from build123d import *

# Parameters (mm, degrees)
SKETCH_1_W          = 50
SKETCH_1_H          = 30
EXTRUDE_1_DEPTH     = 15
SKETCH_2_W          = 19
SKETCH_2_H          = 11.7
CUT_EXTRUDE_1_DEPTH = 28
SKETCH_4_W          = 7.5
SKETCH_4_H          = 13
CUT_EXTRUDE_3_DEPTH = 50
SKETCH_5_W          = 7.5
SKETCH_5_H          = 13
CUT_EXTRUDE_4_DEPTH = 50
CUT_EXTRUDE_5_DEPTH = 50


with BuildPart() as part:
    # Эскиз1 → Бобышка-Вытянуть1 (new body)
    with BuildSketch(Plane.XY):
        Rectangle(SKETCH_1_W, SKETCH_1_H)
    extrude(amount=EXTRUDE_1_DEPTH)

    # Эскиз2 → Вырез-Вытянуть1 (cut)
    with BuildSketch(Plane(origin=(0, 15, 0), x_dir=(1, 0, 0), z_dir=(0, 1, 0))):
        with Locations((0, -9.15)):
            Rectangle(SKETCH_2_W, SKETCH_2_H)
    extrude(amount=-CUT_EXTRUDE_1_DEPTH, mode=Mode.SUBTRACT)

    # Эскиз4 → Вырез-Вытянуть3 (cut)
    with BuildSketch(Plane(origin=(0, 15, 0), x_dir=(1, 0, 0), z_dir=(0, 1, 0))):
        with Locations((-21.25, -6.5)):
            Rectangle(SKETCH_4_W, SKETCH_4_H)
    extrude(amount=-CUT_EXTRUDE_3_DEPTH, mode=Mode.SUBTRACT)

    # Эскиз5 → Вырез-Вытянуть4 (cut)
    with BuildSketch(Plane(origin=(0, 15, 0), x_dir=(1, 0, 0), z_dir=(0, 1, 0))):
        with Locations((21.25, -6.5)):
            Rectangle(SKETCH_5_W, SKETCH_5_H)
    extrude(amount=-CUT_EXTRUDE_4_DEPTH, mode=Mode.SUBTRACT)

    # Эскиз6 → Вырез-Вытянуть5 (cut)
    with BuildSketch(Plane.XZ.offset(15)):
        with BuildLine():
            Line((-5, 15), (5, 15))
            ThreePointArc((5, 15), (0, 10), (-5, 15))
        make_face()
    extrude(amount=-CUT_EXTRUDE_5_DEPTH, mode=Mode.SUBTRACT)


solid = part.part
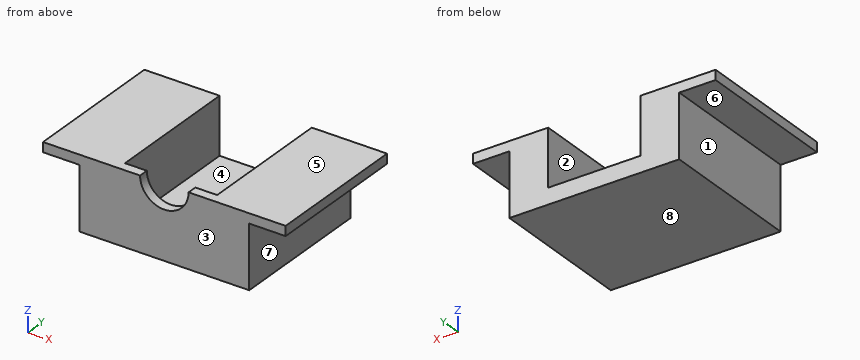
Here's how the part is built. I have some questions about the finished solid (model axes, mm). Face numbers are marked on the shaded views. A direction names the side the tool comes from. Coordinates: 2 decimals unless noted, no trailing zeros. Loops run counter-clockwise (first coordinate to the right, second up) from the corner with the lowest first, then second, coordinate; pieces in that order, holes last. Notation, with made-up numbers: (10.5, 36) -> (26.5, 36) arc R8 ccw to (26.5, 41) -> close; hole circle Ø4 at (-2.75, -4.5). An arc over 180 degrees is marked (long way). Use one line per item in the form item = value. Start each with the question number.
(1) If we section it at A-A (z = 9.25): Please give me the cut outline in (x, y).
(2) Please list where these lines run through material, in increasing order: line 1 along X through (y, z) = (4, 7); line 2 along Y through (x, z) = (6, 13.5); line 3 along Z through (x, y) = (2.5, -3.75).
(3) If we section it at B-B (x = 6): Please give me the cut outline in (y, z).
(4) We'd pull the mould along X, two halves only. Please class the marked faces 1, 2 and 3: pulls with the +X half, pulls with the -X half, needs draft (parallel to the pull), parting line crosses it, or undercut.
(5) Will these pins go through, and if not, where does the flat tip stop? pin 1 (9.5 mm diameter, centred on x = 2.5, y = 4, fed in from +Z); pin 2 (4 mm diameter, centred on x = -22, y = -3, fed in from -Z).
(6) If we section it at D-D (x = 0): Please give me the cut outline in (y, z), then the cut area to 3 significant figures.
(7) On a 3-axis mill with a long thin cutter (end or side, diameter ignored), from which of +Z, -Z, +X, -X, +Y, -Y can I reach the whole of each face in a straight line? I mean the marked faces 4, 5, 6, 7 and 8. Say none if no direction works.
(8) If we section it at C-C (y = -8.5): Please give me the cut outline in (x, z), then the cut area to 3 significant figures.
Verdict:
q1.outline = (-17.5, -15) -> (17.5, -15) -> (17.5, 15) -> (9.5, 15) -> (9.5, -13) -> (-9.5, -13) -> (-9.5, 15) -> (-17.5, 15) -> close
q2.line_1 = -17.5 to -9.5, 9.5 to 17.5
q2.line_2 = -15 to -13
q2.line_3 = 0 to 3.3
q3.outline = (-15, 0) -> (15, 0) -> (15, 3.3) -> (-13, 3.3) -> (-13, 15) -> (-15, 15) -> close
q4.face_1 = pulls with the -X half
q4.face_2 = undercut
q4.face_3 = needs draft
q5.pin_1 = 3.3
q5.pin_2 = 13
q6.outline = (-15, 0) -> (15, 0) -> (15, 3.3) -> (-13, 3.3) -> (-13, 10) -> (-15, 10) -> close
q6.area = 112 mm²
q7.face_4 = +Z, +Y
q7.face_5 = +Z, +X, -X, +Y, -Y
q7.face_6 = -Z, -X, +Y, -Y
q7.face_7 = -Z, +X, +Y, -Y
q7.face_8 = -Z, +X, -X, +Y, -Y
q8.outline = (-25, 13) -> (-17.5, 13) -> (-17.5, 0) -> (17.5, 0) -> (17.5, 13) -> (25, 13) -> (25, 15) -> (9.5, 15) -> (9.5, 3.3) -> (-9.5, 3.3) -> (-9.5, 15) -> (-25, 15) -> close
q8.area = 333 mm²
